Design review of the part shown in the three views and the two pictorial views. Dimensions are in mm from the part's minimum x, y and z. A direction names the side the tool comes from. Coordinates: 2 decimals unless noted, no trailing zeros. Write each loop counter-clockwise with the first axis right and the second up, starting at its lowest first coordinate (ties: lowest second). Pieces come first, ordered by that corner, then holes. Notation, with made-up numbers: M 44,59.25 L 68,59.25 A27 cw 68,85.25 Z; hole C -25.5,89.25 d7. An arc over 180 degrees is marked long. Answer as a JSON object with one key per item and string values.
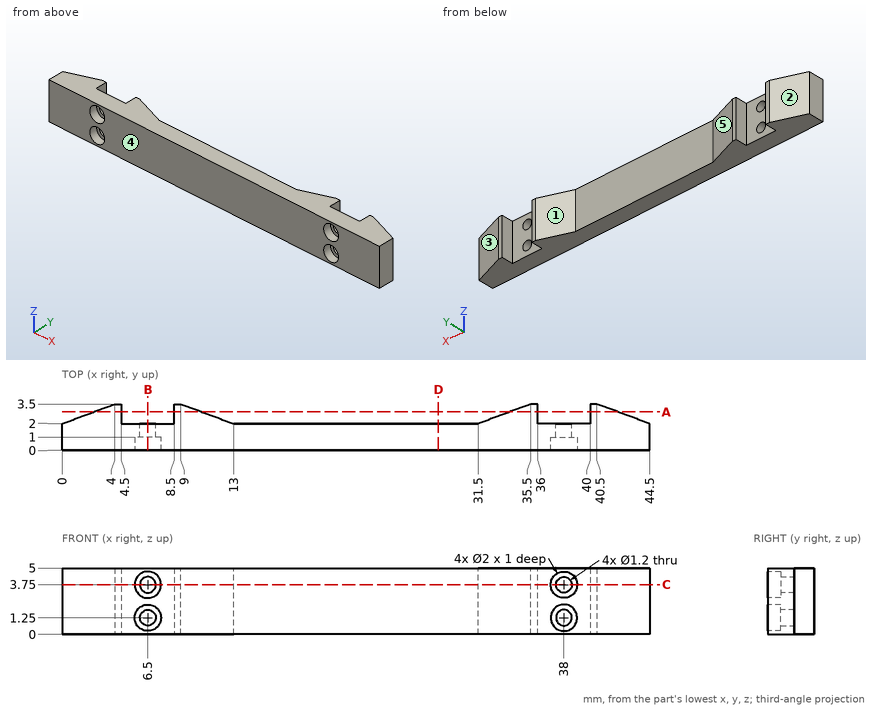
(1) Add section C-C on z = 3.75. Count the separate pieces of the cut face and the enclosed holes in it, and give its area (3 significant figures).
Results list:
{"separate pieces": "3", "enclosed holes": "0", "area": "97.6 mm²"}
(2) Wall thickness on line 1 along Z through (x, y) = (38, 0.55); line 2 along X through (y, z) = (1.5, 1.25); line 3 along Z through (x, y) = (38, 1.7): over which ranges is each line inside the solid? List them lowest first. Write a range as from..to.
Results list:
{"line 1": "0..0.25, 2.25..2.75, 4.75..5", "line 2": "0..5.9, 7.1..37.4, 38.6..44.5", "line 3": "0..0.65, 1.85..3.15, 4.35..5"}
(3) Add section A-A on y = 2.9. Give the boundary of the cut face in (x, z).
Results list:
{"outline": "M 2.4,0 L 4.5,0 L 4.5,5 L 2.4,5 Z; M 8.5,0 L 10.6,0 L 10.6,5 L 8.5,5 Z; M 33.9,0 L 36,0 L 36,5 L 33.9,5 Z; M 40,0 L 42.1,0 L 42.1,5 L 40,5 Z"}
(4) Add section D-D on x = 28.5. Give the boundary of the cut face in (y, z), and give its area (3 significant figures).
Results list:
{"outline": "M 0,0 L 2,0 L 2,5 L 0,5 Z", "area": "10.0 mm²"}
(5) Draft analysis for pull direction X (two halves, no side actions). For the marked faces 1, 2 and 3, state which applies: released by +X, released by -X, zero draft, split by the parting line, or undercut.
Results list:
{"face 1": "undercut", "face 2": "released by -X", "face 3": "released by +X"}
(6) For pin 1 Ø1.6 at (x, z) = (38, 1.25) entering from +Y; pin 2 Ø1 at (x, z) = (38, 1) entering from -Y, all flat-tipped, find the tip position at first contact; note any pin that passes through.
Results list:
{"pin 1": "y = 2", "pin 2": "y = 1"}
(7) For the marked faces 4 and 5, list the 3-axis set-ups (+Z, -Z, +X, -X, +Y, -Y) from which the entire face can be reached by the end or side of a thin tool; tool diameter is ignored.
Results list:
{"face 4": "+Z, -Z, +X, -X, -Y", "face 5": "+Z, -Z, +Y"}
(8) Add section B-B on x = 6.5. Give the boundary of the cut face in (y, z).
Results list:
{"outline": "M 0,0 L 2,0 L 2,0.65 L 1,0.65 L 1,0.25 L 0,0.25 Z; M 0,2.25 L 1,2.25 L 1,1.85 L 2,1.85 L 2,3.15 L 1,3.15 L 1,2.75 L 0,2.75 Z; M 0,4.75 L 1,4.75 L 1,4.35 L 2,4.35 L 2,5 L 0,5 Z"}
